Geometry: final body of the model. Coordinates: model frame, mm. A direction names the side the tool comes from. Coordinates: 2 decimals unless noted, no trailing zeros. Order: outer loops, then holes, each group sorted by start corner. A loop starts at its lowest first (then second) coordinate and runs counter-clockwise, first axis right, second up. Notation, with made-up numbers: M 33.5,43.25 L 51.5,43.25 A24 ccw 51.5,61.25 Z; hole C 14.5,11 d3. An arc over 180 degrees is marked long. Write item = value, one per line. Start each with the question number.
```python
from build123d import *

# Parameters (mm, degrees)
F0_R     = 6.5
F1_DEPTH = 10
F0_R_2   = 9.5
F2_DEPTH = 20


with BuildPart() as f1:
    # F0 (on Front) → F1 (new body)
    with BuildSketch(Plane.XZ):
        with BuildLine():
            ThreePointArc((-13.040623, -13.818182), (-16.353666, 9.672518), (5.828214, 18.084024))
            ThreePointArc((5.828214, 18.084024), (-28.178216, 24.88709), (-62.841564, 23.804848))
            ThreePointArc((-62.841564, 23.804848), (-69.270753, 25.700477), (-72.001132, 31.82199))
            ThreePointArc((-72.001132, 31.82199), (-85.910993, 45.999717), (-100, 32))
            Line((-100, 32), (-100, 18.614531))
            ThreePointArc((-100, 18.614531), (-101.259043, 14.306457), (-104.639875, 11.354396))
            ThreePointArc((-104.639875, 11.354396), (-131.285838, -4.457663), (-154.171786, -25.344547))
            ThreePointArc((-154.171786, -25.344547), (-133.227406, -20.248043), (-121, -38))
            Line((-121, -38), (-121, -70))
            ThreePointArc((-121, -70), (-121.286974, -73.289778), (-122.139225, -76.480179))
            ThreePointArc((-122.139225, -76.480179), (-87.401951, -28.828969), (-32.57725, -7.113346))
            ThreePointArc((-32.57725, -7.113346), (-22.084121, -8.35379), (-13.040623, -13.818182))
        make_face()
        with Locations((-86, 32)):
            Circle(F0_R, mode=Mode.SUBTRACT)
    extrude(amount=F1_DEPTH)

    # F0 (on Front) → F2 (join)
    with BuildSketch(Plane.XZ):
        with BuildLine():
            ThreePointArc((-159, -70), (-143.289778, -88.713026), (-122.139225, -76.480179))
            ThreePointArc((-122.139225, -76.480179), (-121.286974, -73.289778), (-121, -70))
            Line((-121, -70), (-121, -38))
            ThreePointArc((-121, -38), (-133.227406, -20.248043), (-154.171786, -25.344547))
            ThreePointArc((-154.171786, -25.344547), (-157.751957, -31.227406), (-159, -38))
            Line((-159, -38), (-159, -70))
        make_face()
        with BuildLine():
            ThreePointArc((-149.5, -38), (-140, -28.5), (-130.5, -38))
            Line((-130.5, -38), (-130.5, -70))
            ThreePointArc((-130.5, -70), (-140, -79.5), (-149.5, -70))
            Line((-149.5, -70), (-149.5, -38))
        make_face(mode=Mode.SUBTRACT)
        with BuildLine():
            ThreePointArc((-13.040623, -13.818182), (7.524233, -17.446659), (19, 0))
            ThreePointArc((19, 0), (15.357996, 11.18624), (5.828214, 18.084024))
            ThreePointArc((5.828214, 18.084024), (-16.353666, 9.672518), (-13.040623, -13.818182))
        make_face()
        Circle(F0_R_2, mode=Mode.SUBTRACT)
    extrude(amount=F2_DEPTH)


solid = f1.part
```
Item 1: Section query D-D on y = -7.5. Output: boundary loops of the cut face in (x, z), and give its area (3 significant figures).
Item 2: Section query C-C on x = 1.5. Output: boundary loops of the cut face in (y, z).
Item 3: Reachability of faces 1 (the cylindrical face through (-139.791, -9.86, -79.498)), 2 (the flat face through (-121, -15, -54)), 3 (the cylindrical face through (-121.295, -14.93, -73.335)) from +Z, -Z, +X, -X, +Y, -Y: full face, straight path, thin tool, end or side. Return the list, or none.
Item 4: Material intervals for probe 1 along Z at (x, y) = (0, -16); probe 2 along Z at (x, y) = (-86, -3.5); probe 3 along Y at (x, z) = (-79, 0), sorted ascending. Write a range as [from, to].
Item 5: First-contact query: pin 1 (10 mm diameter, centred on y = -11, z = -45.5, fed in from +X); pin 2 (21 mm diameter, centred on x = -86, z = 32, fed in from -Y); pin 3 (6 mm diameter, centred on y = -7, z = 19.5, fed in from +X). Flat tips, straight axial feed; report the tip coordinate or a pass-through.
Item 6: Section query A-A on y = -17.5. Output: boundary loops of the cut face in (x, z).
Item 7: Draft query along Z for faces 4 (the cylindrical face through (4.38, -9.86, -8.43)), 5 (the cylindrical face through (-143.655, -9.86, -88.645)), 6 (the flat face through (-100, -5, 25)). Return one class per face: pulls with the +Z half, pulls with the -Z half, needs draft (parallel to the pull), parting line crosses it, or undercut.
Item 8: Section query B-B on z = -59. Output: boundary loops of the cut face in (x, y).
Ans:
q1.outline = M -159,-70 A19 ccw -122.14,-76.48 A106 cw -32.58,-7.11 A25 cw -13.04,-13.82 A19 ccw long 5.83,18.08 A152 ccw -62.84,23.8 A8 cw -72,31.82 A14 ccw long -100,32 L -100,18.61 A8 cw -104.64,11.35 A152 ccw -154.17,-25.34 A19 ccw -159,-38 Z; hole M -149.5,-70 A9.5 ccw -130.5,-70 L -130.5,-38 A9.5 ccw -149.5,-38 Z; hole C -86,32 d13; hole C 0,0 d19
q1.area = 7,940 mm^2
q2.outline = M -20,-18.94 L 0,-18.94 L 0,-9.38 L -20,-9.38 Z; M -20,9.38 L 0,9.38 L 0,19.41 L -10,19.41 L -10,18.94 L -20,18.94 Z
q3.face_1 = +Y, -Y
q3.face_2 = +Z, -Z, +X, -Y
q3.face_3 = -Z, +X, -Y
q4.probe_1 = [-19, -9.5], [9.5, 19]
q4.probe_2 = [-27.76, 25.5], [38.5, 46]
q4.probe_3 = [-10, 0]
q5.pin_1 = -100.26
q5.pin_2 = -10
q5.pin_3 = 9.42
q6.outline = M -159,-70 A19 ccw -122.14,-76.48 A19 ccw -121,-70 L -121,-38 A19 ccw -159,-38 Z; C 0,0 d38; hole M -149.5,-70 A9.5 ccw -130.5,-70 L -130.5,-38 A9.5 ccw -149.5,-38 Z; hole C 0,0 d19
q7.face_4 = undercut
q7.face_5 = pulls with the -Z half
q7.face_6 = needs draft
q8.outline = M -159,-20 L -149.5,-20 L -149.5,0 L -159,0 Z; M -130.5,-20 L -121,-20 L -121,-10 L -113.93,-10 L -113.93,0 L -130.5,0 Z
